Source: CAD feature listing. Evaluate the final solid. Frame: model axes, mm. A direction names the side the tool comes from. Coordinates: 2 decimals unless noted, no trailing zeros. Loops run counter-clockwise (first coordinate to the right, second up) from the corner with the lowest first, then second, coordinate; pieces in that order, holes last.
Item 1: Line query: probe 1 along X at (y, z) = (-2.5, 1.25); probe 2 along X at (y, z) = (-1.75, 1.45); probe 3 along Y at (x, z) = (-20.5, 1.35). Output: solid intervals per line, ascending.
Item 2: Reachability of faces 1 (the flat face through (-7.25, -2, 2)), 2 (the flat face through (-32, -2.25, 2)), 3 (the flat face through (6.25, -2, 2)) from +Z, -Z, +X, -X, +Y, -Y: full face, straight path, thin tool, end or side. Return the list, or none.
Item 3: Section query B-B, the plane y = 2.75. Return the cut outline in (x, z).
Item 4: Section query D-D, the plane x = -3. Return the cut outline in (y, z), then the cut area to 3 significant figures.
Item 5: Section query C-C, the plane x = -30. Return the cut outline in (y, z), then the cut area to 3 significant figures.
Item 6: Pin query (flat end, axial travel): pin 1 Ø1.1 at (y, z) = (-2, 2) entering from +X; pin 2 Ø1 at (y, z) = (4, 2.5) entering from +X; pin 3 Ø1.5 at (x, z) = (-28, 2) entering from +Y; pin 4 Ø2 at (x, z) = (-19, 2) entering from +Y. Return the tip coordinate at first contact, or that it passes through.
Item 7: Pull-direction query (X, two-part tool) for faces 4 (the cylindrical face through (-32.099, -5.465, 2.028)), 5 (the flat face through (32.4, -3, 2)), 6 (the cylindrical face through (-6.82, -5.15, 2.03)), 7 (the flat face through (32, -2.25, 2)); classes: +X half, -X half, draft (parallel to the pull), parting line (faces both ways), or undercut.
```python
from build123d import *

# Parameters (mm, degrees)
F1_DEPTH = 4
F2_R     = 0.99999
F3_R     = 2
F4_W     = 1.4
F4_H     = 4
F5_DEPTH = 1.5
F6_R     = 1


# Not quite as in the source:
# - a fillet or chamfer is up to 0.001 mm smaller than in the source, because OpenCascade refuses the exact size


with BuildPart() as f1:
    # F0 (on Top) → F1 (new body)
    with BuildSketch(Plane.XY):
        with BuildLine():
            Line((-6.25, -5.75), (-6.25, -3.6742346142))
            ThreePointArc((-6.25, -3.6742346142), (-6.9955342898, -1.9039432765), (-7.25, 0))
            Line((-7.25, 0), (-7.25, -4.75))
            Line((-7.25, -4.75), (-27.6, -4.75))
            Line((-27.6, -4.75), (-27.6, -3.75))
            Line((-27.6, -3.75), (-29, -3.75))
            ThreePointArc((-29, -3.75), (-30, -4.75), (-31, -3.75))
            Line((-31, -3.75), (-32.4, -3.75))
            ThreePointArc((-32.4, -3.75), (-31.6928932188, -4.0428932188), (-31.4, -4.75))
            ThreePointArc((-31.4, -4.75), (-31.6928932188, -5.4571067812), (-32.4, -5.75))
            Line((-32.4, -5.75), (-6.25, -5.75))
        make_face()
        with BuildLine():
            Line((-32.4, -3.75), (-32.4, -5.75))
            ThreePointArc((-32.4, -5.75), (-31.6928932188, -5.4571067812), (-31.4, -4.75))
            ThreePointArc((-31.4, -4.75), (-31.6928932188, -4.0428932188), (-32.4, -3.75))
        make_face()
        with BuildLine():
            ThreePointArc((-6.25, 0), (-4.4194173824, 4.4194173824), (0, 6.25))
            Line((0, 6.25), (0, 7.25))
            ThreePointArc((0, 7.25), (-5.1265241636, 5.1265241636), (-7.25, 0))
            ThreePointArc((-7.25, 0), (-6.9955342898, -1.9039432765), (-6.25, -3.6742346142))
            Line((-6.25, -3.6742346142), (-6.25, 0))
        make_face()
    extrude(amount=F1_DEPTH)

    # F2 (radius 1 in the source; OpenCascade refuses exactly that, so slightly less here)
    f2_edges = [f1.edges().sort_by_distance(p)[0] for p in [
        (-27.6, -4.75, 2),
        (-7.25, -4.75, 2),
    ]]
    fillet(f2_edges, radius=F2_R)

    # F3
    f3_edges = [f1.edges().sort_by_distance(p)[0] for p in [
        (-6.25, -5.75, 2),
    ]]
    fillet(f3_edges, radius=F3_R)

    # F4 (on face) → F5 (join)
    with BuildSketch(Plane(origin=(0, -3.75, 0), x_dir=(-1, 0, 0), z_dir=(0, 1, 0))):
        with Locations((28.3, 2)):
            Rectangle(F4_W, F4_H)
        with Locations((31.7, 2)):
            Rectangle(F4_W, F4_H)
    extrude(amount=F5_DEPTH)

    # F6
    f6_edges = [f1.edges().sort_by_distance(p)[0] for p in [
        (-32.4, -5.75, 2),
    ]]
    fillet(f6_edges, radius=F6_R)

    # F7: F1 across plane


with BuildPart() as f1_1:
    add(f1.part)
    add(f1.part.mirror(Plane.YZ))


solid = f1_1.part
```
Verdict:
1. probe 1: x = -32.4 to -31, -29 to -27.6, -7.25 to -6.25, 6.25 to 7.25, 27.6 to 29, 31 to 32.4
1. probe 2: x = -7.25 to -6.25, 6.25 to 7.25
1. probe 3: y = -5.75 to -4.75
2. face 1: +Z, -Z, +Y
2. face 2: +Z, -Z, -X, +Y
2. face 3: +Z, -Z, -Y
3. outline: (-6.71, 0) - (-5.61, 0) - (-5.61, 4) - (-6.71, 4) - close; (5.61, 0) - (6.71, 0) - (6.71, 4) - (5.61, 4) - close
4. outline: (5.48, 0) - (6.6, 0) - (6.6, 4) - (5.48, 4) - close
4. area: 4.47 mm2
5. outline: (-5.75, 0) - (-4.75, 0) - (-4.75, 4) - (-5.75, 4) - close
5. area: 4.00 mm2
6. pin 1: stops at x = 32.4
6. pin 2: stops at x = 6.35
6. pin 3: stops at y = -2.25
6. pin 4: stops at y = -4.75
7. face 4: -X half
7. face 5: +X half
7. face 6: undercut
7. face 7: draft
